Geometry: final body of the model. Coordinates: model frame, mm. Coordinates: 2 decimals unless noted, no trailing zeros. Loops run counter-clockwise (first coordinate to the right, second up) from the corner with the lowest first, then second, coordinate; pieces in that order, holes last. Notation, with made-up numbers: (80.25, 85.25) - (109.25, 85.25) arc R17 ccw to (109.25, 91.25) - close; hole circle Ø8 at (-37, 60.25). An arc over 180 degrees is marked (long way). Return JSON: item names as keys, results as strings.
from build123d import *

# Parameters (mm, degrees)
SKETCH1_R           = 152.4
SKETCH1_R_2         = 101.6
BOSS_EXTRUDE1_DEPTH = 76.2
BOSS_EXTRUDE3_START = -76.2
BOSS_EXTRUDE3_DEPTH = 76.2
SKETCH7_R           = 12.7
CUT_EXTRUDE2_DEPTH  = 999.889514661
SKETCH8_W           = 63.5
SKETCH8_H           = 127
CUT_EXTRUDE3_DEPTH  = 50.8
SKETCH9_W           = 63.5
SKETCH9_H           = 127
CUT_EXTRUDE5_DEPTH  = 50.8
SKETCH11_R          = 107.95
SKETCH11_R_2        = 101.6
BOSS_EXTRUDE4_DEPTH = 2.54


with BuildPart() as part:
    # Sketch1 → Boss-Extrude1 (new body)
    with BuildSketch(Plane.XY):
        with Locations(Location((0, 0, 0), (0, 0, 180))):
            Circle(SKETCH1_R)
        with Locations(Location((0, 0, 0), (0, 0, 180))):
            Circle(SKETCH1_R_2, mode=Mode.SUBTRACT)
    extrude(amount=BOSS_EXTRUDE1_DEPTH)

    # Sketch2 → Boss-Extrude3 (add)
    with BuildSketch(Plane.XY.offset(76.2).offset(BOSS_EXTRUDE3_START)):
        with BuildLine():
            Line((-958.85, 25.4), (-39.674841602, 147.145054092))
            ThreePointArc((-39.674841602, 147.145054092), (-152.4, 0), (-39.674841602, -147.145054092))
            Line((-39.674841602, -147.145054092), (-958.85, -25.4))
            ThreePointArc((-958.85, -25.4), (-984.25, 0), (-958.85, 25.4))
        make_face()
        with BuildLine():
            Line((39.674841602, 147.145054092), (958.85, 25.4))
            ThreePointArc((958.85, 25.4), (984.25, 0), (958.85, -25.4))
            Line((958.85, -25.4), (39.674841602, -147.145054092))
            ThreePointArc((39.674841602, -147.145054092), (152.4, 0), (39.674841602, 147.145054092))
        make_face()
    extrude(amount=BOSS_EXTRUDE3_DEPTH)

    # Sketch7 → Cut-Extrude2 (cut, through all)
    with BuildSketch(Plane.XY.offset(76.2)):
        with Locations((-958.85, 0)):
            Circle(SKETCH7_R)
        with Locations((958.85, 0)):
            Circle(SKETCH7_R)
    extrude(amount=-CUT_EXTRUDE2_DEPTH, mode=Mode.SUBTRACT)

    # Sketch8 → Cut-Extrude3 (cut)
    with BuildSketch(Plane(origin=(984.25, 0, 0), x_dir=(0, 0, -1), z_dir=(1, 0, 0))):
        with Locations((-38.1, 0)):
            Rectangle(SKETCH8_W, SKETCH8_H)
    extrude(amount=-CUT_EXTRUDE3_DEPTH, mode=Mode.SUBTRACT)

    # Sketch9 → Cut-Extrude5 (cut)
    with BuildSketch(Plane(origin=(-984.25, 0, 0), x_dir=(0, 0, -1), z_dir=(1, 0, 0))):
        with Locations((-38.1, 0)):
            Rectangle(SKETCH9_W, SKETCH9_H)
    extrude(amount=CUT_EXTRUDE5_DEPTH, mode=Mode.SUBTRACT)

    # Sketch11 → Boss-Extrude4 (add)
    with BuildSketch(Plane.XY.offset(76.2)):
        Circle(SKETCH11_R)
        with Locations(Location((0, 0, 0), (0, 0, 180))):
            Circle(SKETCH11_R_2, mode=Mode.SUBTRACT)
    extrude(amount=BOSS_EXTRUDE4_DEPTH)


solid = part.part
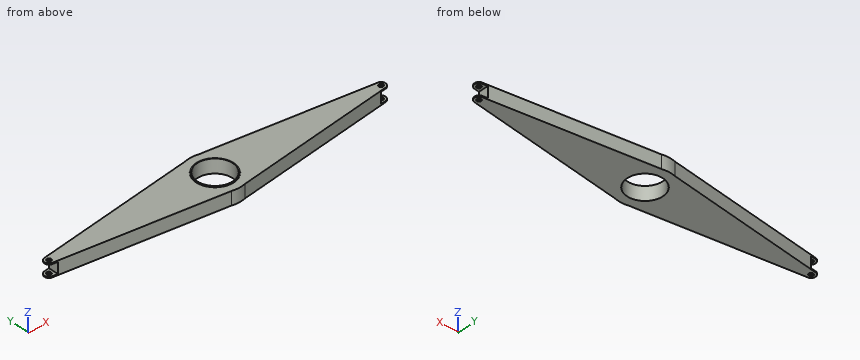
Item 1: First-contact query: pin 1 Ø8 at (x, y) = (398.5, 94) entering from +Z; pin 2 Ø15 at (x, y) = (950, 3) entering from -Z; pin 3 Ø2 at (x, z) = (-198, 44.5) entering from -Y; pin 4 Ø15 at (x, y) = (958.85, 0) entering from +Z. Flat tips, straight axial feed; report the tip coordinate or a pass-through.
Worked out:
{"pin 1": "z = 76.2", "pin 2": "z = 0", "pin 3": "y = -126.31", "pin 4": "through"}
Item 2: Section query D-D, the plane x = 644. Return loops of the section in (y, z).
Worked out:
{"outline": "(-67.1, 0) - (67.1, 0) - (67.1, 76.2) - (-67.1, 76.2) - close"}
Item 3: Section query C-C, the plane x = -211.5. Return loops of the section in (y, z).
Worked out:
{"outline": "(-124.39, 0) - (124.39, 0) - (124.39, 76.2) - (-124.39, 76.2) - close"}
Item 4: Ray query, probe 1 along Y at (x, z) = (958.85, 73); probe 2 along Z at (x, y) = (-104.5, 90.5); probe 3 along Y at (x, z) = (-86, 36). Return the intervals inside material, ascending. Write a range as from..to.
Worked out:
{"probe 1": "-25.4..-12.7, 12.7..25.4", "probe 2": "0..76.2", "probe 3": "-141.01..-54.1, 54.1..141.01"}
Item 5: Section query A-A, the plane x = 0. Return loops of the section in (y, z).
Worked out:
{"outline": "(-152.4, 0) - (-101.6, 0) - (-101.6, 78.74) - (-107.95, 78.74) - (-107.95, 76.2) - (-152.4, 76.2) - close; (101.6, 0) - (152.4, 0) - (152.4, 76.2) - (107.95, 76.2) - (107.95, 78.74) - (101.6, 78.74) - close"}
Item 6: Section query B-B, the plane z = 55. Return loops of the section in (x, y).
Worked out:
{"outline": "(-933.45, -28.76) - (-39.67, -147.15) arc R152.4 ccw to (39.67, -147.15) - (933.45, -28.76) - (933.45, 28.76) - (39.67, 147.15) arc R152.4 ccw to (-39.67, 147.15) - (-933.45, 28.76) - close; hole circle Ø203.2 at (0, 0)"}
